Can you work these out from the model? Positions are in its coordinate system, mm. A direction names the side the tool comes from. Coordinates: 2 decimals unless noted, no trailing zeros. Order: outer loops, then holes, each group sorted by start corner. A loop starts at its lowest first (then second) coordinate and runs counter-clockwise, first axis right, second up. Notation, with made-up numbers: (-18.75, -14.75) -> (-2.75, -14.75) arc R35 cw to (-2.75, 24.25) -> close; hole circle Ø4 at (-19.75, 74). An arc over 180 degrees is marked (long way). Write item = value, one per line. Start each with the question number.
from build123d import *

# Parameters (mm, degrees)
F1_DEPTH = 108.8898
F2_R     = 50.8
F3_R     = 5.08
F5_DEPTH = 635


with BuildPart() as f1:
    # F0 (on Top) → F1 (new body)
    with BuildSketch(Plane.XY):
        Polygon((76.2579515576, 19.2914448351), (-78.5804484424, 19.2914448351), (-78.5804484424, 30.7262744755), (-90.2520939708, 30.7262744755), (-90.2520939708, -14.095553197), (-78.5804484424, -14.095553197), (-78.5804484424, 6.5914448351), (76.2579515576, 6.5914448351), (76.2579515576, -14.095553197), (88.9579515576, -14.095553197), (88.9579515576, 62.104446803), (76.2579515576, 62.104446803), align=None)
    extrude(amount=F1_DEPTH)

    # F2
    f2_edges = [f1.edges().sort_by_distance(p)[0] for p in [
        (82.607952, 62.104447, 108.8898),
        (82.607952, 62.104447, 0),
    ]]
    fillet(f2_edges, radius=F2_R)

    # F3
    f3_edges = [f1.edges().sort_by_distance(p)[0] for p in [
        (-84.416271, 30.726274, 105.030535),
        (-84.416271, 30.726274, 3.859265),
    ]]
    fillet(f3_edges, radius=F3_R)

    # F4 (on Right) → F5 (cut, symmetric)
    with BuildSketch(Plane.YZ):
        with BuildLine():
            ThreePointArc((0, 77.0634550929), (-3.7197438789, 86.043711214), (-12.7, 89.7634550929))
            Line((-12.7, 89.7634550929), (-24.0334216505, 89.7634550929))
            Line((-24.0334216505, 89.7634550929), (-24.0334216505, 17.5617840141))
            Line((-24.0334216505, 17.5617840141), (-12.7, 17.5617840141))
            ThreePointArc((-12.7, 17.5617840141), (-3.7197438789, 21.281527893), (0, 30.2617840141))
            Line((0, 30.2617840141), (0, 77.0634550929))
        make_face()
    extrude(amount=F5_DEPTH, both=True, mode=Mode.SUBTRACT)


solid = f1.part
(1) For faces 1 (the face through (-84.5, 29.74, 104.51)), 2 (the face through (-84.3, -3.8, 21.2)), 3 (the face through (0, 19.291, 54)), 4 (the face through (76.258, 1, 54)), which set-ups out of +Z, -Z, +X, -X, +Y, -Y let a thin tool reach every point of the face, with its end or its side?
(2) Imagine slicing it at C-C (z = 56). Write out the boundary of the cut face in (x, y).
(3) If I drill on L1, parallel to X at y = 2, z = 104.5; L2, parallel to X at y = 31, z = 51; L3, parallel to Y at x = 12, z = 27, over which ranges is the centre line in solid material (lowest first)? Write a range as from..to.
(4) Imagine slicing it at B-B (y = -7). Write out the boundary of the cut face in (x, z), plus the area to 3 significant figures.
(5) For P1, Ø13, axis at x = -85.5, z = 57.5, coming from the +Y side; P2, Ø1.1, axis at x = -82.5, y = -13, coming from the -Z side; P3, Ø4, axis at x = 79.5, z = 59.5, coming from the -Y side; P4, Ø2, axis at x = -30.5, z = 66.5, coming from the +Y side, each with a flat end and sliding along its axis, tell me the tip position at first contact or that it passes through.
(6) Imagine slicing it at D-D (x = 57.5). Write out the boundary of the cut face in (y, z), plus the area to 3 significant figures.
(7) Thinking about a two-plate mould opening in X: for faces 5 (the face through (88.958, 23, 54)), 6 (the face through (-84, -14.096, 99)), 7 (the face through (76.258, 36, 54)), which applies, +X half, -X half, draft (parallel to the pull), parting line (faces both ways), or undercut?
(8) Imagine slicing it at A-A (y = 4). Write out the boundary of the cut face in (x, z).
Result set:
q1.face_1 = +Z, -X, +Y
q1.face_2 = +X, -X, -Y
q1.face_3 = +Z, -Z, +Y
q1.face_4 = +Z, -Z, -Y
q2.outline = (-90.25, 0) -> (-78.58, 0) -> (-78.58, 6.59) -> (76.26, 6.59) -> (76.26, 0) -> (88.96, 0) -> (88.96, 62.1) -> (76.26, 62.1) -> (76.26, 19.29) -> (-78.58, 19.29) -> (-78.58, 30.73) -> (-90.25, 30.73) -> close
q3.L1 = -90.25..-78.58, 76.26..88.96
q3.L2 = 76.26..88.96
q3.L3 = 6.59..19.29
q4.outline = (-90.25, 0) -> (-78.58, 0) -> (-78.58, 18.91) -> (-90.25, 18.91) -> close; (-90.25, 88.41) -> (-78.58, 88.41) -> (-78.58, 108.89) -> (-90.25, 108.89) -> close; (76.26, 0) -> (88.96, 0) -> (88.96, 18.91) -> (76.26, 18.91) -> close; (76.26, 88.41) -> (88.96, 88.41) -> (88.96, 108.89) -> (76.26, 108.89) -> close
q4.area = 960 mm2
q5.P1 = 30.73
q5.P2 = 0
q5.P3 = 0
q5.P4 = 19.29
q6.outline = (6.59, 0) -> (11.3, 0) arc R50.8 ccw to (19.29, 0.63) -> (19.29, 108.26) arc R50.8 ccw to (11.3, 108.89) -> (6.59, 108.89) -> close
q6.area = 1,380 mm2
q7.face_5 = +X half
q7.face_6 = draft
q7.face_7 = undercut
q8.outline = (-90.25, 0) -> (-78.58, 0) -> (-78.58, 108.89) -> (-90.25, 108.89) -> close; (76.26, 0) -> (88.96, 0) -> (88.96, 108.89) -> (76.26, 108.89) -> close
